The figure shows three views and two pictorial views of one solid part (mm, origin at its lowest corner). Answer the questions. A direction names the side the tool comes from. Give positions to 0.01 mm unless a question says otherwise; leave off trailing zeros. Order: outer loops, then holes, each group sorted by start corner. A loop starts at its lowest first (then second) coordinate and runs counter-clockwise, first axis right, second up. Notation, with made-up numbers: (4.5, 78.5) - (19.5, 78.5) arc R21 ccw to (19.5, 99.5) - close; hole circle Ø1 at (54, 89). An arc over 180 degrees is marked (long way). Answer as CSV lines item,"result". Start each with the question number.
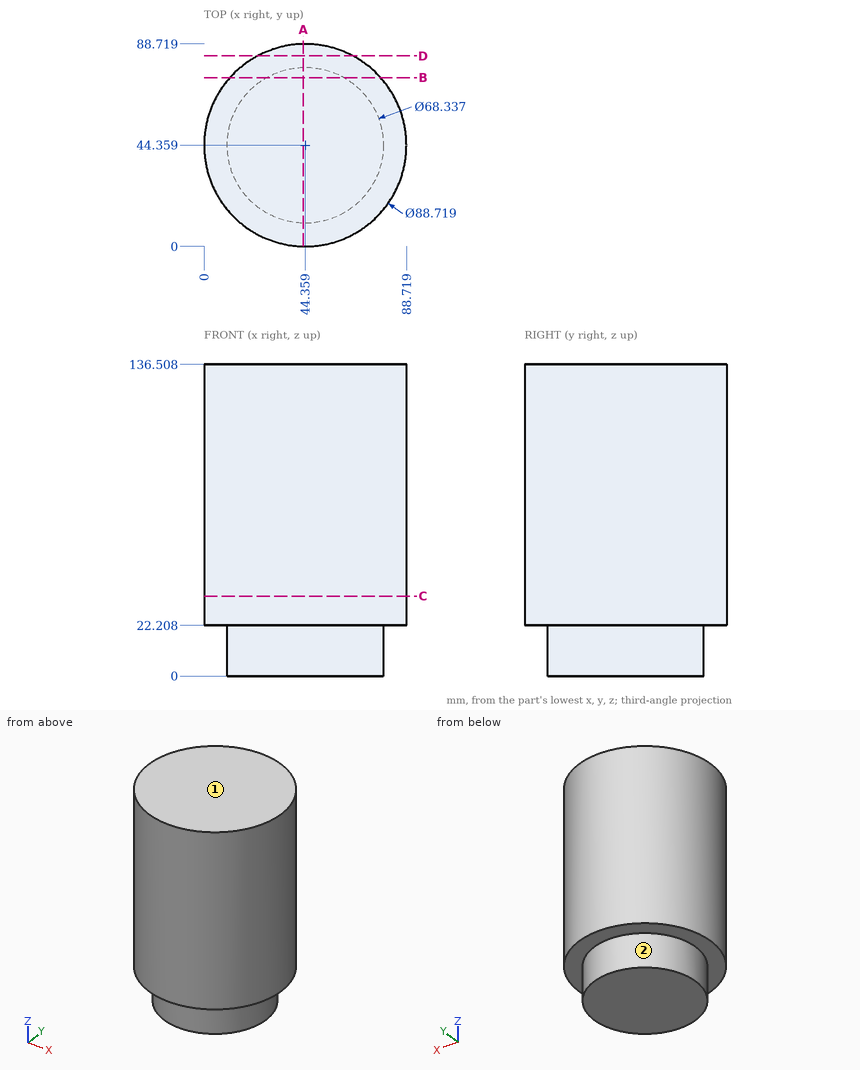
(1) Section C-C, the plane z = 35 is taken. Write down the section's boundary in (x, y).
(2) Section A-A, the plane x = 43.5 is taken. Write down the section's boundary in (y, z).
(3) Section D-D, the plane y = 83.5 is taken. Write down the section's boundary in (x, z) (1 decimal).
(4) Which of the six approach directions +Z, -Z, +X, -X, +Y, -Y give full straight-line access (tool end or side, diameter ignored) to the marked faces 1 and 2?
(5) Straight lines are drawn through the part: line 1 (Z direction, x = 60, y = 9); line 2 (X direction, y = 45, z = 127) (1 decimal); line 3 (X direction, y = 63, z = 113). For each, find the intervals that lie inside material, in ascending order. Write a range as [from, to].
(6) Flat-ended cylindrical pins translate along their axes: pin 1 Ø6 at (x, z) = (9, 97) entering from -Y; pin 2 Ø8 at (x, z) = (40.5, 105) entering from +Y; pin 3 Ø10 at (y, z) = (42.5, 38) entering from -X; pin 4 Ø5 at (y, z) = (76.5, 92.5) entering from -X. Find the tip coordinate at first contact, or state that the pin passes through.
(7) Section B-B, the plane y = 74 is taken. Write down the section's boundary in (x, z), and give its area (3 significant figures).
Checks:
1,outline,"circle Ø88.72 at (44.36, 44.36)"
2,outline,"(0.01, 22.21) - (10.2, 22.21) - (10.2, 0) - (78.52, 0) - (78.52, 22.21) - (88.71, 22.21) - (88.71, 136.51) - (0.01, 136.51) - close"
3,outline,"(23.5, 22.2) - (65.2, 22.2) - (65.2, 136.5) - (23.5, 136.5) - close"
4,face 1,"+Z, +X, -X, +Y, -Y"
4,face 2,"-Z"
5,line 1,"z = [22.21, 136.51]"
5,line 2,"x = [0, 88.7]"
5,line 3,"x = [4.11, 84.61]"
6,pin 1,"stops at y = 14.02"
6,pin 2,"stops at y = 88.72"
6,pin 3,"stops at x = 0"
6,pin 4,"stops at x = 11.36"
7,outline,"(11.36, 22.21) - (27.36, 22.21) - (27.36, 0) - (61.36, 0) - (61.36, 22.21) - (77.36, 22.21) - (77.36, 136.51) - (11.36, 136.51) - close"
7,area,"8,300 mm²"
